Autodesk Inventor part; units mm, degrees
ref_plane "YZ Plane" through (0, 0, 0) normal (1, 0, 0) x (0, 1, 0)
ref_plane "XZ Plane" through (0, 0, 0) normal (0, 1, 0) x (-1, 0, 0)
ref_plane "XY Plane" through (0, 0, 0) normal (0, 0, 1) x (1, 0, 0)
sketch "Skizze1" plane through (0, 0, 0) normal (0, 1, 0) x (-1, 0, 0)
  line L0 (-27, 27) -> (27, 27)
  line L1 (27, 27) -> (27, -27)
  line L2 (27, -27) -> (-27, -27)
  line L3 (-27, -27) -> (-27, 27)
  line L4 (-27, 27) -> (27, -27) construction
  line L5 (27, 27) -> (-27, -27) construction
  point P0 (0, 0)
  dimension "d0" = 54
  dimension "d1" = 54
extrude "Extrusion1" add sketch "Skizze1" along normal blind 3
chamfer "Fase1" distance 2 angle 45 4 edges at (27, 1.5, 27) (27, 1.5, -27) (-27, 1.5, 27) (-27, 1.5, -27)
sketch "Skizze2" plane through (0, 3, 0) normal (0, 1, 0) x (1, 0, 0)
  circle A0 centre (0, 0) radius 11
  dimension "d7" = 22
extrude "Extrusion2" [suppressed]
sketch "Skizze4" plane through (0, 3, 0) normal (0, 1, 0) x (1, 0, 0)
  line L0 (-24, -24) -> (24, -24)
  line L1 (24, -24) -> (24, 24)
  line L2 (24, 24) -> (-24, 24)
  line L3 (-24, 24) -> (-24, -24)
  line L4 (-24, -24) -> (24, 24) construction
  line L5 (24, -24) -> (-24, 24) construction
  point P0 (0, 0)
  dimension "d13" = 48
  dimension "d14" = 48
hole "Bohrung1" at (24, 3, -24) at (24, 3, 24) at (-24, 3, 24) at (-24, 3, -24) direction (0, -1, 0) diameter 3.4 end through all
sketch "Skizze5" plane through (0, 0, 0) normal (0, -1, 0) x (1, 0, 0)
  line L0 (15, 37) -> (-15, 37)
  line L1 (-15, 37) -> (-15, 17)
  line L2 (-15, 17) -> (15, 17)
  line L3 (15, 17) -> (15, 37)
  line L4 (-25, 27) -> (25, 27)
  line L5 (15, 37) -> (-15, 17) construction
  line L6 (-15, 37) -> (15, 17) construction
  point P0 (0, 0)
  point P1 (0, 27)
  dimension "d22" = 30
  dimension "d23" = 10
extrude "Extrusion4" cut sketch "Skizze5" against normal blind 3
fillet "Rundung1" radius 2 2 edges at (-15, 1.5, 17) (15, 1.5, 17)
properties part number "bearing_mount_part_1" material "Aluminium 6061"
Geometry check sheet. Reference: the model listing, model coordinates, mm. A direction names the side the tool comes from. Coordinates: 2 decimals unless noted, no trailing zeros. Loops run counter-clockwise (first coordinate to the right, second up) from the corner with the lowest first, then second, coordinate; pieces in that order, holes last. Notation, with made-up numbers: (32.25, -5) -> (44.25, -5) arc R27 ccw to (44.25, 33) -> close; hole circle Ø5 at (-25.5, 20). An arc over 180 degrees is marked (long way). Put each result on its own line as item: value.
1) Cross-section at B-B on y = 1.6. Record the boundary of the cut face in (x, z), plus the area to 3 significant figures.
Result set:
outline: (-27, -25) -> (-25, -27) -> (25, -27) -> (27, -25) -> (27, 25) -> (25, 27) -> (15, 27) -> (15, 19) arc R2 cw to (13, 17) -> (-13, 17) arc R2 cw to (-15, 19) -> (-15, 27) -> (-25, 27) -> (-27, 25) -> close; hole circle Ø3.4 at (-24, -24); hole circle Ø3.4 at (-24, 24); hole circle Ø3.4 at (24, -24); hole circle Ø3.4 at (24, 24)
area: 2,570 mm^2
2) Tool access check on faces 5 (the cylindrical face through (14.43, 1.52, 17.6)), 6 (the flat face through (26, 2, 26)). Record the directions out of +Z, -Z, +X, -X, +Y, -Y that give a thin tool (end or side, any length) a straight path to the whole face; none if there is none.
Result set:
face 5: +Z, +Y, -Y
face 6: +Z, +X, +Y, -Y
3) Thickness scan on line 1 (Z direction, x = 24, y = 0.8); line 2 (X direction, y = 0.95, z = 24). Record the ranges inside material, lowest first.
Result set:
line 1: z = -27 to -25.7, -22.3 to 22.3, 25.7 to 27
line 2: x = -27 to -25.7, -22.3 to -15, 15 to 22.3, 25.7 to 27
4) Cross-section at A-A on z = 24. Record the boundary of the cut face in (x, y).
Result set:
outline: (-27, 0) -> (-25.7, 0) -> (-25.7, 3) -> (-27, 3) -> close; (-22.3, 0) -> (-15, 0) -> (-15, 3) -> (-22.3, 3) -> close; (15, 0) -> (22.3, 0) -> (22.3, 3) -> (15, 3) -> close; (25.7, 0) -> (27, 0) -> (27, 3) -> (25.7, 3) -> close
5) Cross-section at C-C on z = -24. Record the boundary of the cut face in (x, y).
Result set:
outline: (-27, 0) -> (-25.7, 0) -> (-25.7, 3) -> (-27, 3) -> close; (-22.3, 0) -> (22.3, 0) -> (22.3, 3) -> (-22.3, 3) -> close; (25.7, 0) -> (27, 0) -> (27, 3) -> (25.7, 3) -> close
6) Gauge pin test, flat ends, axial feed: pin 1 Ø10 at (x, z) = (-3.5, 19) entering from +Y; pin 2 Ø1.5 at (x, y) = (-4, 1) entering from +Z. Record the tip position at first contact, or that the pin passes through.
Result set:
pin 1: stops at y = 3
pin 2: stops at z = 17
7) Release check for a two-part mould opening along Z. For faces 1 (the cylindrical face through (22.567, 1.479, -23.086)), 2 (the flat face through (27, 1, 0)), 3 (the cylindrical face through (-25.433, 1.479, -23.086)), 4 (the flat face through (0, 1, -27)) record: released by +Z, released by -Z, zero draft, split by the parting line, or undercut.
Result set:
face 1: undercut
face 2: zero draft
face 3: undercut
face 4: released by -Z
8) Cross-section at D-D on x = -24. Record the boundary of the cut face in (y, z), plus the area to 3 significant figures.
Result set:
outline: (0, -27) -> (3, -27) -> (3, -25.7) -> (0, -25.7) -> close; (0, -22.3) -> (3, -22.3) -> (3, 22.3) -> (0, 22.3) -> close; (0, 25.7) -> (3, 25.7) -> (3, 27) -> (0, 27) -> close
area: 142 mm^2
